The model under review builds one solid part; all positions refer to its coordinate system, in mm. A direction names the side the tool comes from. Give positions to 0.01 mm unless a question says otherwise; leave off trailing zeros. Order: outer loops, then holes, each group sorted by start corner. A loop starts at its lowest first (then second) coordinate and runs counter-clockwise, first axis right, second up.
Autodesk Fusion 360 part; units mm, degrees
sketch "Sketch1" plane through (0, 0, 0) normal (0, 0, 1) x (1, 0, 0)
  circle A0 centre (0, 0) radius 3.25
  circle A1 centre (0, 0) radius 4.75
  circle A2 centre (0, 0) radius 6.35
  dimension "d1" = 6.5
  dimension "d2" = 9.5
  dimension "d3" = 12.7
extrude "Extrude1" add sketch "Sketch1" along normal blind 1.2 contours A2
extrude "Extrude2" add sketch "Sketch1" along normal blind 13.6 contours A1
extrude "Extrude3" cut 1 faces at (4.2202, -0.3974, 13.6) along direction (0, 0, -1) blind 1.2
Item 1: Draft analysis for pull direction X (two halves, no side actions). For faces 1 (the cylindrical face through (-2.579, 1.978, 6.113)), 2 (the flat face through (1, -5, 1.2)), 3 (the cylindrical face through (-1.38, 6.2, 0.59)), state which applies: released by +X, released by -X, zero draft, split by the parting line, or undercut.
Values found:
face 1: undercut
face 2: zero draft
face 3: split by the parting line
Item 2: For faces 4 (the cylindrical face through (2.192, 4.214, 6.722)), 5 (the flat face through (-3, 2, 0)), list the 3-axis set-ups (+Z, -Z, +X, -X, +Y, -Y) from which the entire face can be reached by the end or side of a thin tool; tool diameter is ignored.
Values found:
face 4: +Z
face 5: -Z, +X, -X, +Y, -Y
Item 3: Take a section at A-A (y = 0). Give the boundary of the cut face in (x, z), and give its area (3 significant figures).
Values found:
outline: (-6.35, 0) - (-3.25, 0) - (-3.25, 12.4) - (-4.75, 12.4) - (-4.75, 1.2) - (-6.35, 1.2) - close; (3.25, 0) - (6.35, 0) - (6.35, 1.2) - (4.75, 1.2) - (4.75, 12.4) - (3.25, 12.4) - close
area: 41.0 mm2
Item 4: Clearance check with flat-ended pins moving along their axes: pin 1 Ø3 at (x, z) = (-1, 6) entering from +Y; pin 2 Ø2 at (y, z) = (5, 6.5) entering from -X; pin 3 Ø6 at (y, z) = (-5, 6) entering from -X. State where each tip first meets the part, or that it passes through.
Values found:
pin 1: stops at y = 4.75
pin 2: stops at x = -2.56
pin 3: stops at x = -4.31
Item 5: Take a section at D-D (x = 3.75). Give the boundary of the cut face in (y, z).
Values found:
outline: (-5.12, 0) - (5.12, 0) - (5.12, 1.2) - (2.92, 1.2) - (2.92, 12.4) - (-2.92, 12.4) - (-2.92, 1.2) - (-5.12, 1.2) - close
Item 6: For line 1 (Y direction, x = 0, z = 5.75); line 2 (Z direction, x = 0.25, y = 5); line 3 (X direction, y = 0.25, z = 7.25), list the stretches that pass through material, from the lowest coordinate up.
Values found:
line 1: y = -4.75 to -3.25, 3.25 to 4.75
line 2: z = 0 to 1.2
line 3: x = -4.74 to -3.24, 3.24 to 4.74
Item 7: Take a section at C-C (z = 2). Give the boundary of the cut face in (x, y), and give its area (3 significant figures).
Values found:
outline: circle Ø9.5 at (0, 0); hole circle Ø6.5 at (0, 0)
area: 37.7 mm2
